```python
from build123d import *

# Parameters (mm, degrees)
SKETCH1_W           = 120
SKETCH1_H           = 60
BOSS_EXTRUDE1_DEPTH = 6
SKETCH2_W           = 60
SKETCH2_H           = 100
BOSS_EXTRUDE2_DEPTH = 6
BOSS_EXTRUDE3_DEPTH = 3
SKETCH5_R           = 4
CUT_EXTRUDE2_DEPTH  = 62
SKETCH6_R           = 4
CUT_EXTRUDE3_DEPTH  = 62
FILLET1_R           = 2
FILLET3_R           = 6.5


with BuildPart() as part:
    # Sketch1 → Boss-Extrude1 (new body)
    with BuildSketch(Plane(origin=(0, 0, 0), x_dir=(0, 1, 0), z_dir=(0, 0, 1))):
        Rectangle(SKETCH1_W, SKETCH1_H)
    extrude(amount=BOSS_EXTRUDE1_DEPTH)

    # Sketch2 → Boss-Extrude2 (add)
    with BuildSketch(Plane(origin=(0, 60, 0), x_dir=(-1, 0, 0), z_dir=(0, 1, 0))):
        with Locations((0, 56)):
            Rectangle(SKETCH2_W, SKETCH2_H)
    extrude(amount=-BOSS_EXTRUDE2_DEPTH)

    # Sketch4 → Boss-Extrude3 (add, symmetric)
    with BuildSketch(Plane.YZ):
        Polygon((54, 6), (4, 6), (54, 56), align=None)
    extrude(amount=BOSS_EXTRUDE3_DEPTH, both=True)

    # Sketch5 → Cut-Extrude2 (cut)
    with BuildSketch(Plane(origin=(0, 60, 0), x_dir=(-1, 0, 0), z_dir=(0, 1, 0))):
        with Locations((-15, 81)):
            Circle(SKETCH5_R)
        with Locations((15, 81)):
            Circle(SKETCH5_R)
    extrude(amount=-CUT_EXTRUDE2_DEPTH, mode=Mode.SUBTRACT)

    # Sketch6 → Cut-Extrude3 (cut)
    with BuildSketch(Plane.XY.offset(6)):
        with Locations((-15, -45)):
            Circle(SKETCH6_R)
        with Locations((15, -45)):
            Circle(SKETCH6_R)
        with Locations((-15, 39)):
            Circle(SKETCH6_R)
        with Locations((15, 39)):
            Circle(SKETCH6_R)
    extrude(amount=-CUT_EXTRUDE3_DEPTH, mode=Mode.SUBTRACT)

    # Fillet1
    fillet1_edges = [part.edges().sort_by_distance(p)[0] for p in [
        (-3, 54, 31),
        (-3, 29, 6),
        (3, 54, 31),
        (3, 29, 6),
    ]]
    fillet(fillet1_edges, radius=FILLET1_R)

    # Fillet3
    fillet3_edges = [part.edges().sort_by_distance(p)[0] for p in [
        (0, 4, 6),
        (0, 54, 56),
    ]]
    fillet(fillet3_edges, radius=FILLET3_R)


solid = part.part
```
Verification items for the finished model (mm, model axes). A direction names the side the tool comes from. Round coordinates to 2 decimals unless told otherwise and drop trailing zeros. Write each loop counter-clockwise with the first axis right and the second up, starting at its lowest first coordinate (ties: lowest second). Pieces come first, ordered by that corner, then holes. Notation, with made-up numbers: (67, 15.25) -> (114, 15.25) arc R24 ccw to (114, 53.25) -> close; hole circle Ø2 at (16, -0.5). An arc over 180 degrees is marked (long way). Write each question's results on one line, items separated by ' | '.
Q1. Go/stop test with flat-tipped pins: pin 1 Ø18 at (x, z) = (-7, 42.5) entering from -Y; pin 2 Ø6.5 at (x, y) = (-15, 39) entering from +Z; pin 3 Ø1.5 at (x, y) = (13, 47.5) entering from +Z; pin 4 Ø5 at (x, z) = (14, 79) entering from -Y. Record where each tip stops, or that it passes through.
Derived:
pin 1: stops at y = 32.44 | pin 2: passes through | pin 3: stops at z = 6 | pin 4: stops at y = 54
Q2. Draft check along Y on faces 1 (the face through (0, 57, 106)), 2 (the face through (-17.95, 41.7, 3.04)), 3 (the face through (0.07, 53.49, 56.17)). Enter one of: released by +Y, released by -Y, zero draft, split by the parting line, or undercut.
Derived:
face 1: zero draft | face 2: undercut | face 3: released by -Y
Q3. Sectioned sample at A-A, the plane y = 39. Record the boundary of the cut face in (x, z).
Derived:
outline: (-30, 0) -> (-19, 0) -> (-19, 6) -> (-30, 6) -> close; (-11, 0) -> (11, 0) -> (11, 6) -> (5, 6) arc R2 cw to (3, 8) -> (3, 41) -> (-3, 41) -> (-3, 8) arc R2 cw to (-5, 6) -> (-11, 6) -> close; (19, 0) -> (30, 0) -> (30, 6) -> (19, 6) -> close
Q4. Access from +Z, -Z, +X, -X, +Y, -Y to the whole of each face (thin tool, end or side, straight path). Record for faces 4 (the face through (14.479, -41.034, 3.042)), 5 (the face through (3, 40, 21)), 6 (the face through (-3, 40, 21)), 7 (the face through (0, -4, 6)).
Derived:
face 4: +Z, -Z | face 5: +Z, +X, -Y | face 6: +Z, -X, -Y | face 7: +Z, -Y
Q5. Sectioned sample at B-B, the plane z = 81. Record the boundary of the cut face in (x, y).
Derived:
outline: (-30, 54) -> (-19, 54) -> (-19, 60) -> (-30, 60) -> close; (-11, 54) -> (11, 54) -> (11, 60) -> (-11, 60) -> close; (19, 54) -> (30, 54) -> (30, 60) -> (19, 60) -> close
Q6. Sectioned sample at D-D, the plane z = 16. Record the boundary of the cut face in (x, y).
Derived:
outline: (-30, 54) -> (-5, 54) arc R2 cw to (-3, 52) -> (-3, 14) -> (3, 14) -> (3, 52) arc R2 cw to (5, 54) -> (30, 54) -> (30, 60) -> (-30, 60) -> close
Q7. Sectioned sample at C-C, the plane x = 15. Record the boundary of the cut face in (y, z), and give its area (3 significant figures).
Derived:
outline: (-60, 0) -> (-49, 0) -> (-49, 6) -> (-60, 6) -> close; (-41, 0) -> (35, 0) -> (35, 6) -> (-41, 6) -> close; (43, 0) -> (60, 0) -> (60, 77) -> (54, 77) -> (54, 6) -> (43, 6) -> close; (54, 85) -> (60, 85) -> (60, 106) -> (54, 106) -> close | area: 1,180 mm²
Q8. Thickness scan on probe 1 along Y at (x, z) = (15, 2.4); probe 2 along Z at (x, y) = (15, 58.25); probe 3 along Y at (x, z) = (5, 33). Record the ranges inside material, lowest first.
Derived:
probe 1: y = -60 to -49, -41 to 35, 43 to 60 | probe 2: z = 0 to 77, 85 to 106 | probe 3: y = 54 to 60
